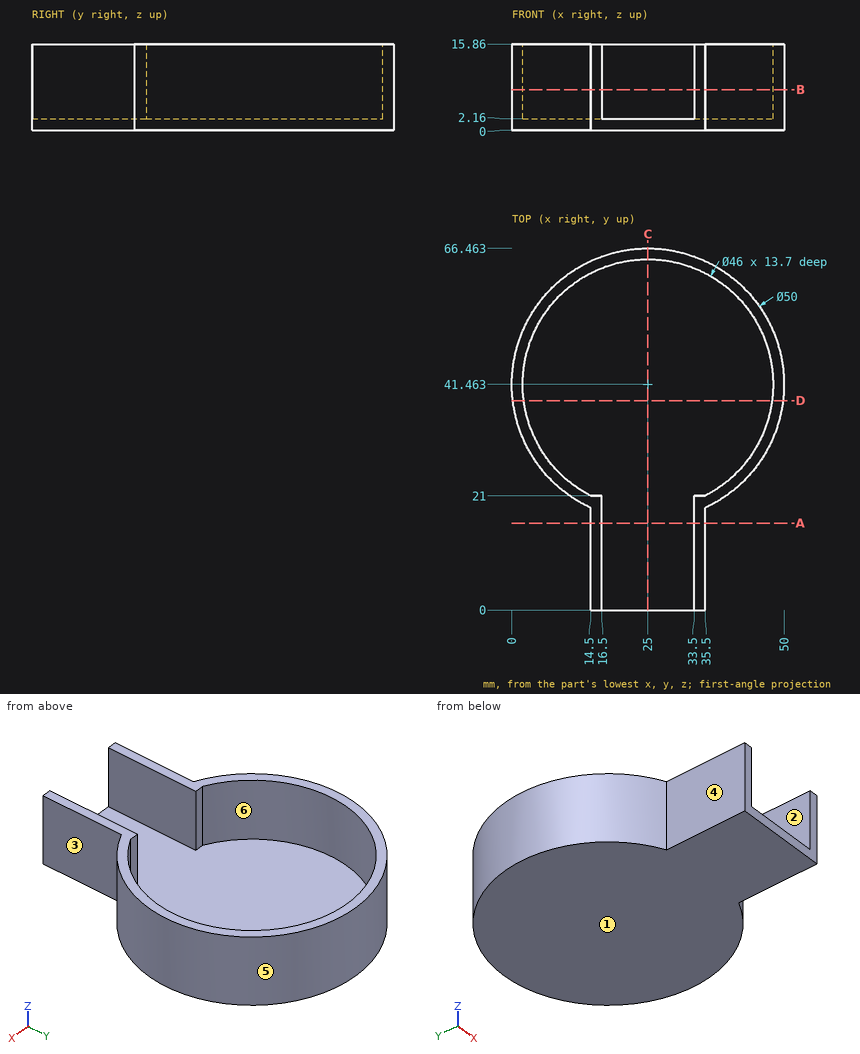
Part print with two shaded views. Sizes in mm from the minimum x, y, z corner. A direction names the side the tool comes from. Coordinates: 2 decimals unless noted, no trailing zeros. Write each loop counter-clockwise with the first axis right and the second up, starting at its lowest first coordinate (ties: lowest second). Pieces come first, ordered by that corner, then holes.
(1) Cut at A-A on y = 16. List the corners of the cut face in (x, z), and give its area (3 significant figures).
(2) Cut at B-B on z = 7.5. List the corners of the cut face in (x, y) (1 decimal).
(3) Cut at C-C on x = 25. List the corners of the cut face in (y, z).
(4) 3-axis set-ups, long thin cutter, end or side, ignore diameter. For the marked faces 1, 2 and 3: which of +Z, -Z, +X, -X, +Y, -Y reach the whole face in a straight line?
(5) Pin check, flat tips, straight feed: pin 1 Ø1 at (y, z) = (54, 4) entering from +X; pin 2 Ø3 at (y, z) = (52, 14) entering from +X; pin 3 Ø0.6 at (x, z) = (34, 8.5) entering from +Y. Stop position of each tip, or through.
(6) Mould opens along X. For the marked faces 4, 5 and 6 say: pulls with the +X half, pulls with the -X half, needs draft (parallel to the pull), parting line crosses it, or undercut.
(7) Cut at D-D on y = 38.5. List the corners of the cut face in (x, z).
(8) Drill centre lines: line 1 (X direction, y = 4, z = 4.5); line 2 (Z direction, x = 11.5, y = 51); line 3 (Y direction, x = 38, z = 10.5). Where is each one in solid material? Low to high.
Working result:
1. outline: (14.5, 0) - (35.5, 0) - (35.5, 15.86) - (33.5, 15.86) - (33.5, 2.16) - (16.5, 2.16) - (16.5, 15.86) - (14.5, 15.86) - close
1. area: 100 mm2
2. outline: (14.5, 0) - (16.5, 0) - (16.5, 21) - (14.5, 21) arc R23 cw (long way) to (35.5, 21) - (33.5, 21) - (33.5, 0) - (35.5, 0) - (35.5, 18.8) arc R25 ccw (long way) to (14.5, 18.8) - close
3. outline: (0, 0) - (66.46, 0) - (66.46, 15.86) - (64.46, 15.86) - (64.46, 2.16) - (0, 2.16) - close
4. face 1: -Z, +X, -X, +Y, -Y
4. face 2: +Z, -Y
4. face 3: +Z, -Z, +X, -Y
5. pin 1: stops at x = 46.91
5. pin 2: stops at x = 48.31
5. pin 3: stops at y = 64.9
6. face 4: pulls with the -X half
6. face 5: parting line crosses it
6. face 6: undercut
7. outline: (0.18, 0) - (49.82, 0) - (49.82, 15.86) - (47.81, 15.86) - (47.81, 2.16) - (2.19, 2.16) - (2.19, 15.86) - (0.18, 15.86) - close
8. line 1: x = 14.5 to 16.5, 33.5 to 35.5
8. line 2: z = 0 to 2.16
8. line 3: y = 20.11 to 22.49, 60.44 to 62.82
